Geometry: final body of the model. Coordinates: model frame, mm. A direction names the side the tool comes from. Coordinates: 2 decimals unless noted, no trailing zeros. Write each loop counter-clockwise with the first axis right and the second up, starting at its lowest first coordinate (ties: lowest second). Pieces come first, ordered by that corner, then holes. Notation, with made-up numbers: (-32, 30) -> (24, 30) arc R3 ccw to (24, 35) -> close; hole circle Ø7 at (40.25, -6.5). An arc over 180 degrees is marked (long way). One line per item, written item: value.
```python
from build123d import *

# Parameters (mm, degrees)
SKETCH1_R             = 84.1375
SKETCH1_R_2           = 1.8288
BOSS_EXTRUDE1_DEPTH   = 4.7625
CIRPATTERN1_OUTLINE_R = 1.8288
CIRPATTERN1_DEPTH     = 4.7625
SKETCH4_R             = 5.588
CUT_EXTRUDE1_DEPTH    = 1.905
CIRPATTERN2_COUNT     = 3


# Read off the part's stored shape, not the designer's step: CirPattern1
with BuildPart() as part:
    # Sketch1 → Boss-Extrude1 (new body)
    with BuildSketch(Plane(origin=(0, 0, 0), x_dir=(1, 0, 0), z_dir=(0, 1, 0))):
        with Locations(Location((0, 0, 0), (0, 0, 90))):
            Circle(SKETCH1_R)
        with BuildLine():
            ThreePointArc((-13.335, -62.213928537), (0, 63.627), (13.335, -62.213928537))
            Line((13.335, -62.213928537), (13.335, -67.437))
            Line((13.335, -67.437), (-13.335, -67.437))
            Line((-13.335, -67.437), (-13.335, -62.213928537))
        make_face(mode=Mode.SUBTRACT)
        with Locations(Location((0, -77.7875, 0), (0, 0, 90))):
            Circle(SKETCH1_R_2, mode=Mode.SUBTRACT)
    extrude(amount=BOSS_EXTRUDE1_DEPTH)

    # CirPattern1 outline → CirPattern1 (cut)
    with BuildSketch(Plane(origin=(0, 0, 0), x_dir=(1, 0, 0), z_dir=(0, 1, 0))):
        with BuildLine():
            Line((65.069655155, -22.170051241), (60.546342582, -19.558515509))
            ThreePointArc((60.546342582, -19.558515509), (55.102598367, -31.8135), (47.211342582, -42.655413028))
            Line((47.211342582, -42.655413028), (51.734655155, -45.266948759))
            Line((51.734655155, -45.266948759), (65.069655155, -22.170051241))
        make_face()
        with BuildLine():
            Line((51.734655155, 45.266948759), (47.211342582, 42.655413028))
            ThreePointArc((47.211342582, 42.655413028), (55.102598367, 31.8135), (60.546342582, 19.558515509))
            Line((60.546342582, 19.558515509), (65.069655155, 22.170051241))
            Line((65.069655155, 22.170051241), (51.734655155, 45.266948759))
        make_face()
        with BuildLine():
            Line((-13.335, 67.437), (-13.335, 62.213928537))
            ThreePointArc((-13.335, 62.213928537), (0, 63.627), (13.335, 62.213928537))
            Line((13.335, 62.213928537), (13.335, 67.437))
            Line((13.335, 67.437), (-13.335, 67.437))
        make_face()
        with BuildLine():
            Line((-65.069655155, 22.170051241), (-60.546342582, 19.558515509))
            ThreePointArc((-60.546342582, 19.558515509), (-55.102598367, 31.8135), (-47.211342582, 42.655413028))
            Line((-47.211342582, 42.655413028), (-51.734655155, 45.266948759))
            Line((-51.734655155, 45.266948759), (-65.069655155, 22.170051241))
        make_face()
        with BuildLine():
            Line((-65.069655155, -22.170051241), (-51.734655155, -45.266948759))
            Line((-51.734655155, -45.266948759), (-47.211342582, -42.655413028))
            ThreePointArc((-47.211342582, -42.655413028), (-55.102598367, -31.8135), (-60.546342582, -19.558515509))
            Line((-60.546342582, -19.558515509), (-65.069655155, -22.170051241))
        make_face()
        with Locations((-67.365951097, -38.89375)):
            Circle(CIRPATTERN1_OUTLINE_R)
        with Locations((-67.365951097, 38.89375)):
            Circle(CIRPATTERN1_OUTLINE_R)
        with Locations((0, 77.7875)):
            Circle(CIRPATTERN1_OUTLINE_R)
        with Locations((67.365951097, 38.89375)):
            Circle(CIRPATTERN1_OUTLINE_R)
        with Locations((67.365951097, -38.89375)):
            Circle(CIRPATTERN1_OUTLINE_R)
    extrude(amount=CIRPATTERN1_DEPTH, mode=Mode.SUBTRACT)

    # Sketch4 → Cut-Extrude1 (cut)
    with BuildSketch(Plane.XZ):
        with Locations(Location((35.40125, -61.316763651, 0), (0, 0, 270))):
            Circle(SKETCH4_R)
    cut_extrude1 = extrude(amount=-CUT_EXTRUDE1_DEPTH, mode=Mode.SUBTRACT)

    # CirPattern2: Cut-Extrude1 ×3 about axis
    cirpattern2_axis = Axis((0, 0, 0), (0, 1, 0))
    for i in range(1, CIRPATTERN2_COUNT):
        add(cut_extrude1.rotate(cirpattern2_axis, i * 360 / CIRPATTERN2_COUNT), mode=Mode.SUBTRACT)


solid = part.part
```
(1) Reachability of faces 3 (the flat face through (-71, 1.905, 0)), 4 (the cylindrical face through (63.626, 2.348, -0.278)) from +Z, -Z, +X, -X, +Y, -Y: full face, straight path, thin tool, end or side. Return the list, or none.
Responses:
face 3: -Y
face 4: +Y, -Y
(2) Pull-direction query (X, two-part tool) for faces 1 (the flat face through (58.31, 2.35, 33.88)), 2 (the flat face through (-32, 0, -56)); classes: released by +X, released by -X, zero draft, split by the parting line, or undercut.
Responses:
face 1: undercut
face 2: zero draft
(3) Line query: line 1 (X direction, y = 2.6, z = -37.5); line 2 (Z direction, x = 2, y = 1.45); line 3 (X direction, y = 1.1, z = -1). Output: solid intervals per line, ascending. Write a range as [from, to].
Responses:
line 1: x = [-75.32, -68.55], [-66.18, -56.22], [56.22, 66.18], [68.55, 75.32]
line 2: z = [-84.11, -67.44], [67.44, 84.11]
line 3: x = [-84.13, -76.3], [-65.3, -63.62], [63.62, 84.13]
(4) Section C-C (y = 3.25). State how many separate pieces and enclosed holes the cut face has, then the cut area to 3 significant figures.
Responses:
separate pieces: 1
enclosed holes: 7
area: 8,770 mm2
(5) Section A-A (z = 0). Return the cut outline in (x, y) (1 decimal), then the cut area to 3 significant figures.
Responses:
outline: (-84.1, 0) -> (-76.4, 0) -> (-76.4, 1.9) -> (-65.2, 1.9) -> (-65.2, 0) -> (-63.6, 0) -> (-63.6, 4.8) -> (-84.1, 4.8) -> close; (63.6, 0) -> (84.1, 0) -> (84.1, 4.8) -> (63.6, 4.8) -> close
area: 174 mm2
(6) Section D-D (x = -10.5). Return the cut outline in (y, z), then the cut area to 3 significant figures.
Responses:
outline: (0, -83.48) -> (4.76, -83.48) -> (4.76, -67.44) -> (0, -67.44) -> close; (0, 67.44) -> (4.76, 67.44) -> (4.76, 83.48) -> (0, 83.48) -> close
area: 153 mm2
(7) First-contact query: pin 1 (5.5 mm diameter, centred on x = 34, z = -59.5, fed in from -Y) (3 decimals); pin 2 (1 mm diameter, centred on y = 2.5, z = -67, fed in from -X); pin 3 (10 mm diameter, centred on x = 37, z = 41.5, fed in from -Y); pin 4 (1.4 mm diameter, centred on x = 6.5, y = 1.5, fed in from -Z). Flat tips, straight axial feed; report the tip coordinate or a pass-through.
Responses:
pin 1: stops at y = 1.905
pin 2: stops at x = -51.54
pin 3: passes through
pin 4: stops at z = -83.94
(8) Section B-B (x = 55.5). Return the cut outline in (y, z).
Responses:
outline: (0, -63.24) -> (4.76, -63.24) -> (4.76, -38.75) -> (0, -38.75) -> close; (0, 38.75) -> (4.76, 38.75) -> (4.76, 63.24) -> (0, 63.24) -> close
